Autodesk Inventor part; units mm, degrees
ref_plane "Work Plane1" through (29, 0, 0) normal (0, -1, 0) x (1, 0, 0)
ref_plane "YZ Plane" through (0, 0, 0) normal (1, 0, 0) x (0, 1, 0)
ref_plane "XZ Plane" through (0, 0, 0) normal (0, 1, 0) x (-1, 0, 0)
sketch "Sketch1" plane through (0, 0, 0) normal (0, 0, 1) x (1, 0, 0)
  line L0 (0.1947, 0) -> (9.525, 0)
  line L1 (9.525, 0) -> (9.525, 3.175)
  line L2 (9.525, 3.175) -> (2.4132, 3.175)
  line L3 (2.4132, 3.175) -> (0.0001, 3.175)
  line L4 (0.0001, 3.175) -> (0, 3.175)
  line L5 (0, 3.175) -> (0, 5.5499)
  line L6 (0, 5.5499) -> (-3.3528, 5.5499)
  line L7 (-3.3528, 5.5499) -> (-3.3528, 2.317)
  line L8 (-3.3528, 2.317) -> (-1.143, 2.317)
  line L9 (-1.143, 2.317) -> (0.1947, 0)
  line L10 (-5.9284, 0) -> (12.1006, 0)
  line L11 (0, -1.11) -> (0, 6.6599)
  line L12 (2.4132, 3.175) -> (0, 3.175) construction
  dimension "d1" = 7.1118
  dimension "d2" = 2.4131
  dimension "d3" = 3.3528
  dimension "d4" = 2.2098
  dimension "d5" = 60
  dimension "d6" = 6.35
  dimension "d7" = 6.35
  dimension "d8" = 4.634
  dimension "d9" = 11.0998
  dimension "d26" = 9.525
revolve "Body" add sketch "Sketch1" angle 360 about axis through (0.1947, 0, 0) along (1, 0, 0) contours L9 L11 L3 L2 L1 L0 | L9 L8 L7 L6 L5 L11
sketch "Sketch2" plane through (-3.3528, 0, 0) normal (-1, 0, 0) x (0, 0, 1)
  circle A0 centre (0, 0) radius 2.317
  line L0 (0, -7.7699) -> (0, 7.7699)
  line L1 (-7.7699, 0) -> (7.7699, 0)
  line L2 (2.317, 0) -> (1.1585, -2.0066)
  line L3 (1.1585, -2.0066) -> (-1.1585, -2.0066)
  line L4 (-1.1585, -2.0066) -> (-2.317, 0)
  line L5 (-2.317, 0) -> (-1.1585, 2.0066)
  line L6 (-1.1585, 2.0066) -> (1.1585, 2.0066)
  line L7 (1.1585, 2.0066) -> (2.317, 0)
extrude "Slot" add sketch "Sketch2" against normal up to next contours L7 A0 | A0 L2 | L6 L0 A0 | A0 L0 L3 | L0 L6 A0 | A0 L3 L0 | L4 A0 | A0 L5
fillet "Fillet1" radius 2.2098 1 edges at (-3.3528, -5.5499, 0)
thread "Thread"
chamfer "Chamfer1" distance 0.7791 distance2 0.779 1 edges at (9.525, -3.175, 0) measured on face at (9.525, 1.7119, 1.0506)
ref_plane "Work Plane1" through (29, 0, 0) normal (0, -1, 0) x (1, 0, 0)
fillet "Fillet2" radius 0.1 1 edges at (0.0001, -3.175, 0)
equation "\"d1\" = GEL"
equation "\"d3\" = KOH"
equation "\"d4\" = INTI"
equation "\"d6\" = GD"
equation "\"d7\" = BDM"
equation "\"d8\" = 1.1547 * SW"
equation "\"d9\" = KOD"
equation "\"d26\" = NLG"
equation "\"d30\" = R"
equation "\"d17\" = RR"
equation "\"d13\" = GEL"
equation "\"d15\" = -0.5 * SPD + 0.5 * GD"
equation "\"d16\" = GUL"
equation "\"GD\" = NND"
equation "\"NLG\" = 9.525"
equation "\"GEL\" = 7.1118"
equation "\"KOD\" = 11.0998"
equation "\"KOH\" = 3.3528"
equation "\"INTI\" = 2.2098"
equation "\"GAL\" = 2.413"
equation "\"GUL\" = 0.77902"
equation "\"BDM\" = NND"
equation "\"SW\" = 4.0132"
equation "\"RR\" = 2.2098"
equation "\"SPD\" = GD1"
equation "\"R\" = 0.1"
equation "\"KR\" = 6.3246"
equation "\"GD1\" = 4.79188"
equation "\"THREADDIA\" = 6.35"
equation "\"FAWI\" = 45deg"
equation "\"KOH1\" = 2.2098"
equation "\"NND\" = 6.35"
equation "\"TOA\" = 30deg"
equation "\"E0\" = 1.155 * SW"
properties part number "Unbrako - 1/4 x 3/8" material "Steel, Mild"
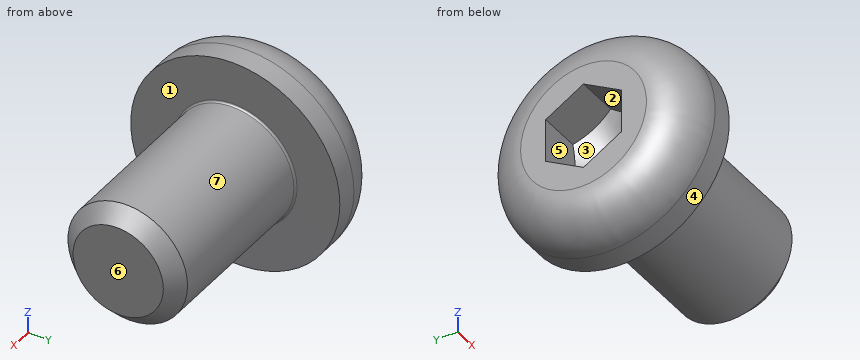
Work out the finished part from the listing and answer in its coordinate system (mm). Face numbers are marked on the shaded views. A direction names the side the tool comes from. Round coordinates to 2 decimals unless told otherwise and drop trailing zeros. Loops run counter-clockwise (first coordinate to the right, second up) from the corner with the lowest first, then second, coordinate; pieces in that order, holes last. Notation, with made-up numbers: M -34,22 L -17,22 A24 cw -17,53 Z; hole C 24,34 d7. An arc over 180 degrees is marked long. One line per question, with ' | ' between items. Start each with the question number.
(1) A tool of negligible diameter and unlimited length cuts with its end or side. For the marked faces 5, 6 and 7, from which of +Z, -Z, +X, -X, +Y, -Y can it reach the whole face along a straight path? Write none if from no direction.
(2) Flat-ended cylindrical pins translate along their axes: pin 1 Ø1.2 at (x, z) = (-1.5, 0) entering from -Y; pin 2 Ø1.5 at (x, y) = (-1, 2.5) entering from -Z; pin 3 Ø2 at (x, z) = (2, -0.5) entering from +Y (3 decimals). Find the tip coordinate at first contact, or state that the pin passes through.
(3) Find the intervals of material crossed by line 1 (Y direction, x = 4, z = 0) (3 decimals); line 2 (Y direction, x = -2.25, z = -2); line 3 (Z direction, x = -0.75, y = 0.5), in increasing order.
(4) For a pull along Y with two mould halves and no side action, classify the marked faces 1, 2, 3 and 4 as released by +Y, released by -Y, zero draft, split by the parting line, or undercut.
(5) A cutting plane is placed at A-A on x = -2.25. Write down the section's boundary in (y, z), plus the area to 3 significant figures.
(6) A cutting plane is placed at B-B on x = 1. Write down the section's boundary in (y, z) (3 decimals).
Geometry check:
1) face 5: -X | face 6: +Z, -Z, +X, +Y, -Y | face 7: +X
2) pin 1: stops at y = -5.55 | pin 2: stops at z = -5.27 | pin 3: stops at y = 3.175
3) line 1: y = -3.175 to 3.175 | line 2: y = -4.86 to -0.55, 0.55 to 4.86 | line 3: z = -5.53 to -1.56, 1.56 to 5.53
4) face 1: zero draft | face 2: undercut | face 3: undercut | face 4: split by the parting line
5) outline: C 0,0 d10.51; hole M -2.01,-1.16 L 0,-2.32 L 2.01,-1.16 L 2.01,1.16 L 0,2.32 L -2.01,1.16 Z | area: 72.7 mm²
6) outline: C 0,0 d6.35
